Geometry check sheet. Reference: the model listing, model coordinates, mm. Face numbers are marked on the shaded views. A direction names the side the tool comes from. Coordinates: 2 decimals unless noted, no trailing zeros. Write each loop counter-clockwise with the first axis right and the second up, starting at its lowest first coordinate (ties: lowest second). Pieces come first, ordered by that corner, then holes. Notation, with made-up numbers: (-8.75, 59) -> (6.25, 59) arc R23 cw to (6.25, 94) -> close; hole circle Ø8 at (-36.5, 58). An arc over 180 degrees is marked (long way). Use a Markdown table: item, result.
Autodesk Fusion 360 part; units mm, degrees
sketch "Sketch1" plane through (0, 0, 0) normal (0, 0, 1) x (1, 0, 0)
  line L0 (0, 0) -> (0, 80)
  line L1 (0, 80) -> (80, 80)
  line L2 (8, 6) -> (8, 68)
  line L3 (12, 72) -> (74, 72)
  line L4 (80, 78) -> (80, 80)
  line L5 (0, 0) -> (2, 0)
  arc A0 (74, 72) -> (80, 78) centre (74, 78) ccw
  arc A1 (2, 0) -> (8, 6) centre (2, 6) ccw
  arc A2 (12, 72) -> (8, 68) centre (12, 68) ccw
  dimension "d1" = 80
  dimension "d2" = 80
  dimension "d4" = 6
  dimension "d5" = 6
  dimension "d6" = 4
extrude "Extrude1" add sketch "Sketch1" along normal mid plane 180
sketch "Sketch2" plane through (0, 0, 0) normal (-1, 0, 0) x (0, 0, 1)
  line L0 (-90, 0) -> (90, 0) construction
  line L1 (90, 0) -> (90, 80) construction
  line L2 (90, 80) -> (-90, 80) construction
  line L3 (-90, 80) -> (-90, 0) construction
  line L4 (-90, 80) -> (90, 80) construction
  line L5 (-90, 0) -> (-90, 80) construction
  line L6 (-90, 0) -> (90, 0) construction
  line L7 (90, 80) -> (90, 0) construction
  line L8 (-90, 40) -> (90, 40) construction
  line L9 (0, 80) -> (0, 0) construction
  circle A0 centre (-65, 40) radius 9
  circle A1 centre (65, 40) radius 9
  dimension "d9" = 18
  dimension "d10" = 65
extrude "Extrude2" cut sketch "Sketch2" against normal through all
sketch "Sketch3" plane through (0, 80, 0) normal (0, 1, 0) x (-1, 0, 0)
  line L0 (0, -90) -> (0, 90) construction
  line L1 (0, 90) -> (-80, 90) construction
  line L2 (-80, 90) -> (-80, -90) construction
  line L3 (-80, -90) -> (0, -90) construction
  line L4 (-80, 90) -> (0, 90) construction
  line L5 (-80, -90) -> (-80, 90) construction
  line L6 (0, -90) -> (0, 90) construction
  line L7 (0, -90) -> (-80, -90) construction
  line L8 (-80, 0) -> (0, 0) construction
  line L9 (-40, -90) -> (-40, 90) construction
  circle A0 centre (-40, -51) radius 9
  circle A1 centre (-40, 51) radius 9
  dimension "d12" = 18
  dimension "d13" = 51
extrude "Extrude3" cut sketch "Sketch3" against normal through all
equation "d13 = ( 102 / 2 ) * 1 mm"
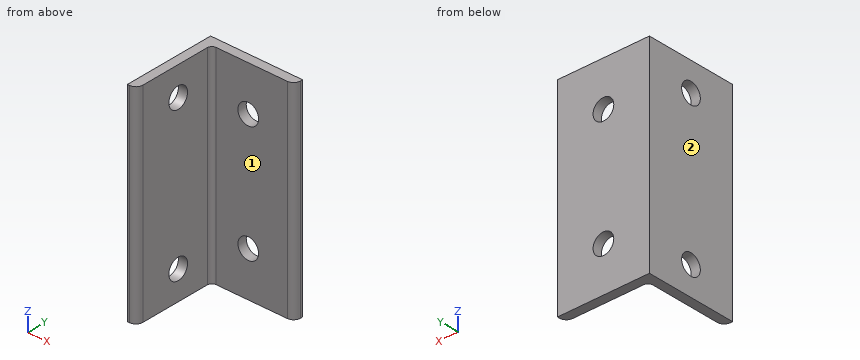
Item 1: Thickness scan on L1, parallel to Y at x = 1, z = 65; L2, parallel to X at y = 47.5, z = -81.5; L3, parallel to Y at x = 14, z = 44. Record the ranges inside material, lowest first. Write a range as [from, to].
Answer block:
| item | result |
|---|---|
| L1 | y = [0, 31], [49, 80] |
| L2 | x = [0, 8] |
| L3 | y = [72, 80] |
Item 2: Depth check by flat-ended pin: P1, Ø16, axis at x = 40, z = 51, coming from the +Y side; P2, Ø6, axis at y = 49, z = 0.5, coming from the +X side; P3, Ø3, axis at x = 64.5, z = 4.5, coming from the -Y side; P4, Ø10, axis at y = 65.5, z = -46.5, coming from the +X side. Enter the tip coordinate at first touch or a pass-through.
Answer block:
| item | result |
|---|---|
| P1 | passes through |
| P2 | stops at x = 8 |
| P3 | stops at y = 72 |
| P4 | stops at x = 8.88 |
Item 3: Section check D-D on x = 56. Record the boundary of the cut face in (y, z).
Answer block:
| item | result |
|---|---|
| outline | (72, -90) -> (80, -90) -> (80, 90) -> (72, 90) -> close |
Item 4: Section check B-B on y = 40. Record the boundary of the cut face in (x, z), then the cut area to 3 significant figures.
Answer block:
| item | result |
|---|---|
| outline | (0, -90) -> (8, -90) -> (8, -74) -> (0, -74) -> close; (0, -56) -> (8, -56) -> (8, 56) -> (0, 56) -> close; (0, 74) -> (8, 74) -> (8, 90) -> (0, 90) -> close |
| area | 1,150 mm^2 |
Item 5: Section check C-C on z = 14. Record the boundary of the cut face in (x, y), then the cut area to 3 significant figures.
Answer block:
| item | result |
|---|---|
| outline | (0, 0) -> (2, 0) arc R6 ccw to (8, 6) -> (8, 68) arc R4 cw to (12, 72) -> (74, 72) arc R6 ccw to (80, 78) -> (80, 80) -> (0, 80) -> close |
| area | 1,200 mm^2 |
Item 6: Section check A-A on z = 65. Record the boundary of the cut face in (x, y).
Answer block:
| item | result |
|---|---|
| outline | (0, 0) -> (2, 0) arc R6 ccw to (8, 6) -> (8, 31) -> (0, 31) -> close; (0, 49) -> (8, 49) -> (8, 68) arc R4 cw to (12, 72) -> (74, 72) arc R6 ccw to (80, 78) -> (80, 80) -> (0, 80) -> close |
Item 7: Tool access check on the marked faces 1 and 2. Record the directions out of +Z, -Z, +X, -X, +Y, -Y that give a thin tool (end or side, any length) a straight path to the whole face; none if there is none.
Answer block:
| item | result |
|---|---|
| face 1 | +Z, -Z, +X, -Y |
| face 2 | +Z, -Z, -X, +Y, -Y |
